Can you work these out from the model? Positions are in its coordinate system, mm. Face numbers are marked on the shaded views. Coordinates: 2 decimals unless noted, no trailing zeros. Order: outer loops, then holes, each group sorted by start corner. A loop starts at its lowest first (then second) coordinate and runs counter-clockwise, first axis right, second up. Notation, with made-up numbers: (-18.75, 27) -> (-4.75, 27) arc R30 ccw to (-4.75, 66) -> close; hole circle Ø10 at (51, 17). An arc over 180 degrees is marked (long way). Write item = value, one per line.
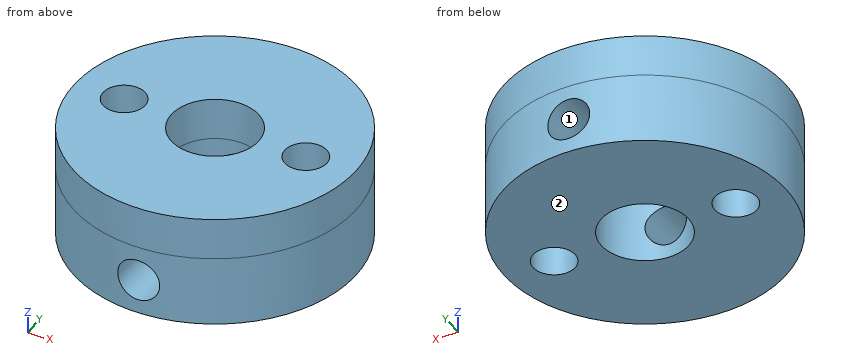
```python
from build123d import *

# Parameters (mm, degrees)
F0_R     = 10
F0_R_2   = 3.1
F1_DEPTH = 2.5
F3_D     = 3
F4_R     = 1.5
F5_DEPTH = 12.5
F6_DEPTH = 3


with BuildPart() as f1:
    # F0 (on Top) → F1 (new body, symmetric)
    with BuildSketch(Plane.XY):
        Circle(F0_R)
        Circle(F0_R_2, mode=Mode.SUBTRACT)
    extrude(amount=F1_DEPTH, both=True)

    # F3 (through all)
    with Locations(Plane.XY.offset(2.5)):
        with Locations((-6.5, 0), (6.5, 0)):
            Hole(F3_D / 2)

    # F4 (on Front) → F5 (cut, symmetric)
    with BuildSketch(Plane.XZ):
        Circle(F4_R)
    extrude(amount=F5_DEPTH, both=True, mode=Mode.SUBTRACT)

    # F6 (add): a face of the model
    f6_faces = [f1.faces().sort_by_distance(p)[0] for p in [
        (-9.7171572875, 0, 2.5),
    ]]
    extrude(f6_faces, amount=F6_DEPTH)


solid = f1.part
```
Item 1: I want a section at B-B, the plane y = 0. Please give me the cut outline in (x, z).
A:
outline = (-10, -2.5) -> (-8, -2.5) -> (-8, 5.5) -> (-10, 5.5) -> close; (-5, -2.5) -> (-3.1, -2.5) -> (-3.1, 5.5) -> (-5, 5.5) -> close; (3.1, -2.5) -> (5, -2.5) -> (5, 5.5) -> (3.1, 5.5) -> close; (8, -2.5) -> (10, -2.5) -> (10, 5.5) -> (8, 5.5) -> close
Item 2: I'm going to push flat-ended pins straight in: P1, Ø2.5, axis at x = 0, z = 0, coming from the -Y side; P2, Ø3, axis at x = 7.5, z = 4.5, coming from the +Y side; P3, Ø2, axis at x = -7, z = -1.5, coming from the -Y side. Where does each tip first touch, or does it pass through?
A:
P1 = through
P2 = 8
P3 = -8
Item 3: I want a section at D-D, the plane y = -2.25. Please give me the cut outline in (x, z), plus the area to 3 significant figures.
A:
outline = (-9.74, -2.5) -> (-2.13, -2.5) -> (-2.13, 5.5) -> (-9.74, 5.5) -> close; (2.13, -2.5) -> (9.74, -2.5) -> (9.74, 5.5) -> (2.13, 5.5) -> close
area = 122 mm2
Item 4: I want a section at C-C, the plane z = 0. Please give me the cut outline in (x, y).
A:
outline = (-1.5, -9.89) -> (-1.5, -2.71) arc R3.1 cw to (-1.5, 2.71) -> (-1.5, 9.89) arc R10 ccw to start; (1.5, -9.89) arc R10 ccw to (1.5, 9.89) -> (1.5, 2.71) arc R3.1 cw to (1.5, -2.71) -> close; hole circle Ø3 at (-6.5, 0); hole circle Ø3 at (6.5, 0)
Item 5: If we mould it in two halves opening along X, with no side actions, what happens to the marked faces 1 and 2? For each: pulls with the +X half, pulls with the -X half, needs draft (parallel to the pull), parting line crosses it, or undercut.
A:
face_1 = undercut
face_2 = needs draft
Item 6: If I drill on probe 1 along Z at (x, y) = (0, 5); probe 2 along X at (y, z) = (-1.25, -0.25); probe 3 along X at (y, z) = (5, -1.25), over which ranges is the centre line in solid material (lowest first)?
A:
probe_1 = -2.5 to -1.5, 1.5 to 5.5
probe_2 = -9.92 to -7.33, -5.67 to -2.84, 2.84 to 5.67, 7.33 to 9.92
probe_3 = -8.66 to -0.83, 0.83 to 8.66
Item 7: I want a section at A-A, the plane x = 0. Please give me the cut outline in (y, z).
A:
outline = (-10, -2.5) -> (-3.1, -2.5) -> (-3.1, -1.5) -> (-10, -1.5) -> close; (-10, 1.5) -> (-3.1, 1.5) -> (-3.1, 5.5) -> (-10, 5.5) -> close; (3.1, -2.5) -> (10, -2.5) -> (10, -1.5) -> (3.1, -1.5) -> close; (3.1, 1.5) -> (10, 1.5) -> (10, 5.5) -> (3.1, 5.5) -> close
